Could you check a few things on this model? Use its own coordinates, in mm. A direction names the side the tool comes from. Give positions to 0.01 mm unless a question says otherwise; leave off trailing zeros. Loops run counter-clockwise (first coordinate to the right, second up) from the corner with the lowest first, then second, coordinate; pieces in that order, holes last.
1. For faces 5 (the flat face through (1, -3, -4)), 6 (the flat face through (2, -3, -5)), 7 (the flat face through (-1, 4.5, 0)), 8 (the flat face through (2, -3, 5)), which set-ups out of +Z, -Z, +X, -X, +Y, -Y let a thin tool reach every point of the face, with its end or its side?
2. Imagine slicing it at B-B (x = 0.25). List the corners of the cut face in (y, z) for me, plus the area to 3 significant figures.
3. Imagine slicing it at C-C (z = 5.25). List the corners of the cut face in (x, y) for me, plus the area to 3 significant figures.
4. Thinking about a two-plate mould opening in Y: for faces 1 (the cylindrical face through (0.139, -2.685, 0.596)), 2 (the flat face through (0, -5.5, 0)), 3 (the cylindrical face through (2, 5, 0)), 4 (the flat face through (-1, -1, -6)), which applies, +Y half, -Y half, draft (parallel to the pull), parting line (faces both ways), or undercut?
5. For P1, Ø0.6, axis at x = 0.5, y = -4, coming from the +Z side; P2, Ø1.9, axis at x = -1.5, z = 2, coming from the +Y side, each with a flat end and sliding along its axis, tell me the tip position at first contact or that it passes through.
6. Imagine slicing it at D-D (x = -1). List the corners of the cut face in (y, z) for me.
7. Imagine slicing it at A-A (z = 0). List the corners of the cut face in (x, y) for me, plus the area to 3 significant figures.
8. I need wall thicknesses on line 1 along X through (y, z) = (2.5, -3.5); line 2 along Y through (x, z) = (0.4, 0); line 3 along Y through (x, z) = (1.4, 0). Which ranges of each line are inside material? Lowest first, please.
```python
from build123d import *

# Parameters (mm, degrees)
BOSS_EXTRUDE1_DEPTH = 1.2
SKETCH2_W           = 12
SKETCH2_H           = 10
BOSS_EXTRUDE2_DEPTH = 3
BOSS_EXTRUDE3_DEPTH = 2
CUT_EXTRUDE1_REACH  = 8.2
SKETCH4_R           = 2.75
FILLET1_R           = 0.3


with BuildPart() as part:
    # Sketch1 → Boss-Extrude1 (new body)
    with BuildSketch(Plane(origin=(0, 0, 0), x_dir=(0, 0, -1), z_dir=(1, 0, 0))):
        with BuildLine():
            Line((-4, 0), (-4, -5.5))
            Line((-4, -5.5), (4, -5.5))
            Line((4, -5.5), (4, 0))
            ThreePointArc((4, 0), (0, 4), (-4, 0))
        make_face()
    extrude(amount=BOSS_EXTRUDE1_DEPTH)

    # Sketch2 → Boss-Extrude2 (add)
    with BuildSketch(Plane.ZY):
        with Locations((0, -0.5)):
            Rectangle(SKETCH2_W, SKETCH2_H)
    extrude(amount=BOSS_EXTRUDE2_DEPTH)

    # Sketch3 → Boss-Extrude3 (add)
    with BuildSketch(Plane(origin=(1.2, 0, 0), x_dir=(0, 0, -1), z_dir=(1, 0, 0))):
        with BuildLine():
            Line((-5, 0), (-5, -5.5))
            Line((-5, -5.5), (5, -5.5))
            Line((5, -5.5), (5, 0))
            ThreePointArc((5, 0), (0, 5), (-5, 0))
        make_face()
    extrude(amount=BOSS_EXTRUDE3_DEPTH)

    # Sketch4 → Cut-Extrude1 (cut, up to next)
    with BuildSketch(Plane(origin=(3.2, 0, 0), x_dir=(0, 0, -1), z_dir=(1, 0, 0)), mode=Mode.PRIVATE) as cut_extrude1_sk1:
        Circle(SKETCH4_R)
    cut_extrude1_tool1 = extrude(cut_extrude1_sk1.sketch, amount=-CUT_EXTRUDE1_REACH, mode=Mode.PRIVATE) & part.part
    add(cut_extrude1_tool1.solids().sort_by_distance((3.2, 0, 0))[0], mode=Mode.SUBTRACT)

    # Fillet1
    fillet1_edges = [part.edges().sort_by_distance(p)[0] for p in [
        (1.2, -2.75, -5),
        (1.2, -2.75, 5),
        (3.2, -2.75, -5),
        (3.2, -2.75, 5),
        (-3, 0, 2.75),
        (-3, 4.5, 0),
        (-1.5, 4.5, -6),
        (-3, -0.5, -6),
        (0, -0.5, -6),
        (0, -5.5, -5),
        (-1.5, -5.5, -6),
        (-3, -5.5, 0),
        (-3, -0.5, 6),
        (0, 4.5, 0),
        (-1.5, 4.5, 6),
        (0, -0.5, 6),
        (-1.5, -5.5, 6),
        (0, -5.5, 5),
        (0.6, -5.5, -4),
        (1.2, -5.5, -4.5),
        (0.6, -5.5, 4),
        (1.2, -5.5, 4.5),
        (2.2, -5.5, -5),
        (2.2, -5.5, 5),
        (1.2, 5, 0),
        (3.2, 0, 2.75),
        (3.2, -5.5, 0),
        (3.2, 5, 0),
    ]]
    fillet(fillet1_edges, radius=FILLET1_R)


solid = part.part
```
Derived:
1. face 5: -Z, +Y, -Y
1. face 6: -Z, +X, +Y, -Y
1. face 7: +Z, -Z, -X, +Y
1. face 8: +Z, +X, +Y, -Y
2. outline: (-5.5, -3.7) arc R0.3 ccw to (-5.2, -4) - (0, -4) arc R4 ccw to (0, 4) - (-5.2, 4) arc R0.3 ccw to (-5.5, 3.7) - close; hole circle Ø5.5 at (0, 0)
2. area: 45.3 mm2
3. outline: (-3, -5.2) arc R0.3 ccw to (-2.7, -5.5) - (-0.3, -5.5) arc R0.3 ccw to (0, -5.2) - (0, 4.2) arc R0.3 ccw to (-0.3, 4.5) - (-2.7, 4.5) arc R0.3 ccw to (-3, 4.2) - close
3. area: 29.9 mm2
4. face 1: undercut
4. face 2: -Y half
4. face 3: +Y half
4. face 4: draft
5. P1: stops at z = 4
5. P2: stops at y = 4.5
6. outline: (-5.5, -5.7) arc R0.3 ccw to (-5.2, -6) - (4.2, -6) arc R0.3 ccw to (4.5, -5.7) - (4.5, 5.7) arc R0.3 ccw to (4.2, 6) - (-5.2, 6) arc R0.3 ccw to (-5.5, 5.7) - close; hole circle Ø5.5 at (0, 0)
7. outline: (-3, -5.2) arc R0.3 ccw to (-2.7, -5.5) - (2.9, -5.5) arc R0.3 ccw to (3.2, -5.2) - (3.2, -3.05) arc R0.3 ccw to (2.9, -2.75) - (-2.7, -2.75) arc R0.3 ccw to (-3, -3.05) - close; (-3, 3.05) arc R0.3 ccw to (-2.7, 2.75) - (2.9, 2.75) arc R0.3 ccw to (3.2, 3.05) - (3.2, 4.7) arc R0.3 ccw to (2.9, 5) - (1.5, 5) arc R0.3 ccw to (1.2, 4.7) - (1.2, 4) - (0, 4) - (0, 4.2) arc R0.3 ccw to (-0.3, 4.5) - (-2.7, 4.5) arc R0.3 ccw to (-3, 4.2) - close
7. area: 28.1 mm2
8. line 1: x = -3 to 0, 1.2 to 3.2
8. line 2: y = -5.5 to -2.75, 2.75 to 4
8. line 3: y = -5.5 to -2.75, 2.75 to 4.98
